Read the model definition and answer for the solid it produces. Units are mm, in the model's axes. Give positions to 0.01 mm unless a question says otherwise; leave off trailing zeros. Write each loop counter-clockwise with the first axis right and the second up, starting at its lowest first coordinate (ties: lowest second). Pieces come first, ordered by that corner, then holes. Notation, with made-up numbers: (78.5, 27) -> (132.5, 27) arc R23 ccw to (132.5, 46) -> close; hole circle Ø6 at (61.5, 29). An arc over 180 degrees is marked (long way). Answer as CSV lines item,"result". Start each with the question number.
1. The part is cut by section C-C, the plane y = 2.6. Determine the outline of the cut face in (x, z), and give its area (3 significant figures).
2. The part is cut by section A-A, the plane x = -19.5. Determine the outline of the cut face in (y, z).
3. Find the intervals of material crossed by line 1 (Z direction, x = -26, y = 3.7); line 2 (Y direction, x = 24, z = -23); line 3 (X direction, y = 2.7, z = -12), in increasing order.
4. Given pin 1 (0.6 mm diameter, centred on x = 18.5, y = 3, fed in from -Z); pin 2 (0.8 mm diameter, centred on y = 0.5, z = 0.5, fed in from -X); pin 3 (1.6 mm diameter, centred on y = 3.5, z = 5, fed in from -X), each flat-ended and moving along its own axis, determine where each tip first touches the part or whether it passes through.
5. The part is cut by section B-B, the plane z = 11. Determine the outline of the cut face in (x, y).
6. The part is cut by section D-D, the plane x = 77. Determine the outline of the cut face in (y, z).
from build123d import *

# Parameters (mm, degrees)
SKETCH1_W           = 160
SKETCH1_H           = 55
BOSS_EXTRUDE1_DEPTH = 2
SKETCH2_W           = 109
SKETCH2_H           = 42
BOSS_EXTRUDE2_DEPTH = 2
CUT_EXTRUDE1_DEPTH  = 2


with BuildPart() as part:
    # Sketch1 → Boss-Extrude1 (new body)
    with BuildSketch(Plane(origin=(0, 0, 0), x_dir=(1, 0, 0), z_dir=(0, 1, 0))):
        with Locations((21.028856201, -0.390930324)):
            Rectangle(SKETCH1_W, SKETCH1_H)
    extrude(amount=BOSS_EXTRUDE1_DEPTH)

    # Sketch2 → Boss-Extrude2 (add)
    with BuildSketch(Plane(origin=(0, 2, 0), x_dir=(1, 0, 0), z_dir=(0, 1, 0))):
        with Locations((21.028856201, -0.390930324)):
            Rectangle(SKETCH2_W, SKETCH2_H)
    extrude(amount=BOSS_EXTRUDE2_DEPTH)

    # Sketch3 → Cut-Extrude1 (cut)
    with BuildSketch(Plane(origin=(0, 2, 0), x_dir=(1, 0, 0), z_dir=(0, 1, 0))):
        with BuildLine():
            Line((-58.971143799, 2.109069676), (-55.971143799, 2.109069676))
            ThreePointArc((-55.971143799, 2.109069676), (-54.556930237, 1.523283239), (-53.971143799, 0.109069676))
            Line((-53.971143799, 0.109069676), (-53.971143799, -0.890930324))
            ThreePointArc((-53.971143799, -0.890930324), (-54.556930237, -2.305143886), (-55.971143799, -2.890930324))
            Line((-55.971143799, -2.890930324), (-58.971143799, -2.890930324))
            Line((-58.971143799, -2.890930324), (-58.971143799, 2.109069676))
        make_face()
        with BuildLine():
            Line((101.028856201, 2.109069676), (98.028856201, 2.109069676))
            ThreePointArc((98.028856201, 2.109069676), (96.614642638, 1.523283239), (96.028856201, 0.109069676))
            Line((96.028856201, 0.109069676), (96.028856201, -0.890930324))
            ThreePointArc((96.028856201, -0.890930324), (96.614642638, -2.305143886), (98.028856201, -2.890930324))
            Line((98.028856201, -2.890930324), (101.028856201, -2.890930324))
            Line((101.028856201, -2.890930324), (101.028856201, 2.109069676))
        make_face()
    extrude(amount=-CUT_EXTRUDE1_DEPTH, mode=Mode.SUBTRACT)


solid = part.part
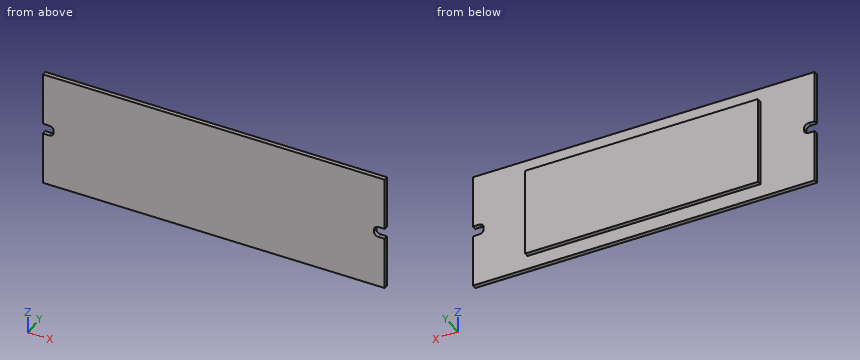
Results found:
1,outline,"(-33.47, -20.61) -> (75.53, -20.61) -> (75.53, 21.39) -> (-33.47, 21.39) -> close"
1,area,"4,580 mm²"
2,outline,"(0, -27.11) -> (2, -27.11) -> (2, -20.61) -> (4, -20.61) -> (4, 21.39) -> (2, 21.39) -> (2, 27.89) -> (0, 27.89) -> close"
3,line 1,"z = -20.61 to 21.39"
3,line 2,"y = 0 to 2"
3,line 3,"x = -33.47 to 75.53"
4,pin 1,"stops at z = -20.61"
4,pin 2,"stops at x = -53.97"
4,pin 3,"stops at x = -33.47"
5,outline,"(-58.97, 0) -> (101.03, 0) -> (101.03, 2) -> (75.53, 2) -> (75.53, 4) -> (-33.47, 4) -> (-33.47, 2) -> (-58.97, 2) -> close"
6,outline,"(0, -27.11) -> (2, -27.11) -> (2, 27.89) -> (0, 27.89) -> close"
